Autodesk Inventor part; units mm, degrees
ref_plane "Work Plane1" through (34.8, 0, 0) normal (1, 0, 0) x (0, 1, 0)
ref_plane "YZ Plane" through (0, 0, 0) normal (1, 0, 0) x (0, 1, 0)
ref_plane "XZ Plane" through (0, 0, 0) normal (0, 1, 0) x (-1, 0, 0)
sketch "Sketch1" plane through (0, 0, 0) normal (0, 0, 1) x (1, 0, 0)
  circle A0 centre (0, 0) radius 19.05
  circle A1 centre (0, 0) radius 17.4
  dimension "d0" = 38.1
  dimension "d3" = 1.65
extrude "Extrusion1" add sketch "Sketch1" along normal blind 120.4
ref_plane "Work Plane1" through (34.8, 0, 0) normal (1, 0, 0) x (0, 1, 0)
sketch "Sketch2" plane through (34.8, 0, 0) normal (1, 0, 0) x (0, 1, 0)
  line L0 (-19.05, 120.4) -> (19.05, 120.4)
  line L1 (-19.05, 0) -> (19.05, 0)
  line L2 (19.05, 0) -> (19.05, 120.4)
  line L3 (-19.05, 0) -> (-19.05, 120.4)
  line L4 (0, 120.4) -> (0, 0) construction
  circle A0 centre (0, 60.2) radius 19.05
  circle A1 centre (0, 60.2) radius 17.4
  dimension "d7" = 38.1
  dimension "d8" = 1.65
extrude "Extrusion2" add sketch "Sketch2" against normal up to next contours A0
sketch "Sketch6" plane through (34.8, 0, 60.2) normal (1, 0, 0) x (0, 0, -1)
  circle A0 centre (0, 0) radius 17.4
  circle A1 centre (0, 0) radius 19.05
  circle A2 centre (0, 0) radius 25.15
  dimension "d17" = 0
  dimension "d18" = 50.3
extrude "Extrusion4" add sketch "Sketch6" against normal blind 3 contours A2
chamfer "Chamfer2" distance 2 angle 45 1 edges at (31.8, 0, 85.35)
properties part number "ASME BPE Eq Inst Tee-38.1"
Geometry: final body of the model. Coordinates: model frame, mm. A direction names the side the tool comes from. Round coordinates to 2 decimals unless told otherwise and drop trailing zeros. Write each loop counter-clockwise with the first axis right and the second up, starting at its lowest first coordinate (ties: lowest second). Pieces come first, ordered by that corner, then holes. Notation, with made-up numbers: (-20.5, -22.5) -> (-7.5, -22.5) arc R21 ccw to (-7.5, -17.5) -> close; hole circle Ø4 at (56, 49). An arc over 180 degrees is marked (long way). Return JSON: item names as keys, results as strings.
Q1. Section B-B on x = 10. Return the cut outline in (y, z).
From the geometry:
{"outline": "(-16.21, 0) -> (-14.24, 0) -> (-14.24, 120.4) -> (-16.21, 120.4) -> (-16.21, 70.2) arc R19.05 ccw to (-16.21, 50.2) -> close; (14.24, 0) -> (16.21, 0) -> (16.21, 50.2) arc R19.05 ccw to (16.21, 70.2) -> (16.21, 120.4) -> (14.24, 120.4) -> close; hole (-16.21, 53.89) -> (-16.21, 66.51) arc R17.4 ccw to start; hole (16.21, 53.89) arc R17.4 ccw to (16.21, 66.51) -> close"}
Q2. Set-up query: faces 4 (the cylindrical face through (34.31, 7.55, 36.21)), 5 (the cylindrical face through (19.66, -19.03, 61.04)), 6 (the cylindrical face through (-3.772, 16.986, 59.357)). Return all of +Z, -Z, +X, -X, +Y, -Y with unobstructed straight access to the full face (end or side cutting, diameter ignored); none if empty.
From the geometry:
{"face 4": "+X", "face 5": "none", "face 6": "+Z, -Z"}
Q3. Mould query, pull axis Y, two halves, no side actions, for faces 1 (the cylindrical face through (-19.03, -0.84, 59.36)), 2 (the flat face through (34.8, 17, 55)), 3 (the cylindrical face through (24.47, 16.597, 65.426)). Classes: +Y half, -Y half, draft (parallel to the pull), parting line (faces both ways), or undercut.
From the geometry:
{"face 1": "parting line", "face 2": "draft", "face 3": "undercut"}
Q4. First-contact query: pin 1 Ø3 at (x, z) = (18.5, 65.5) entering from -Y; pin 2 Ø1 at (x, z) = (15.5, 22) entering from -Y; pin 3 Ø2 at (x, z) = (11, 94.5) entering from -Y; pin 4 Ø12 at (y, z) = (-3, 85.5) entering from +X. Flat tips, straight axial feed; report the tip coordinate or a pass-through.
From the geometry:
{"pin 1": "y = -18.67", "pin 2": "y = -11.74", "pin 3": "y = -16.21", "pin 4": "x = 34.8"}
Q5. Section C-C on x = -12. Return the cut outline in (y, z).
From the geometry:
{"outline": "(-14.8, 0) -> (-12.6, 0) -> (-12.6, 120.4) -> (-14.8, 120.4) -> close; (12.6, 0) -> (14.8, 0) -> (14.8, 120.4) -> (12.6, 120.4) -> close"}
Q6. Section A-A on y = 0. Return the cut outline in (x, z).
From the geometry:
{"outline": "(-19.05, 0) -> (-17.4, 0) -> (-17.4, 120.4) -> (-19.05, 120.4) -> close; (17.4, 0) -> (19.05, 0) -> (19.05, 41.15) -> (31.8, 41.15) -> (31.8, 37.05) -> (33.8, 35.05) -> (34.8, 35.05) -> (34.8, 42.8) -> (19.05, 42.8) -> (19.05, 77.6) -> (34.8, 77.6) -> (34.8, 85.35) -> (33.8, 85.35) -> (31.8, 83.35) -> (31.8, 79.25) -> (19.05, 79.25) -> (19.05, 120.4) -> (17.4, 120.4) -> close"}
Q7. Ray query, line 1 (X direction, y = -0.5, z = 39.5); line 2 (Y direction, x = 0, z = 29.5); line 3 (Z direction, x = 23.25, y = 0). Return the intervals inside material, ascending.
From the geometry:
{"line 1": "-19.04 to -17.39, 17.39 to 19.04, 31.8 to 34.8", "line 2": "-19.05 to -17.4, 17.4 to 19.05", "line 3": "41.15 to 42.8, 77.6 to 79.25"}
